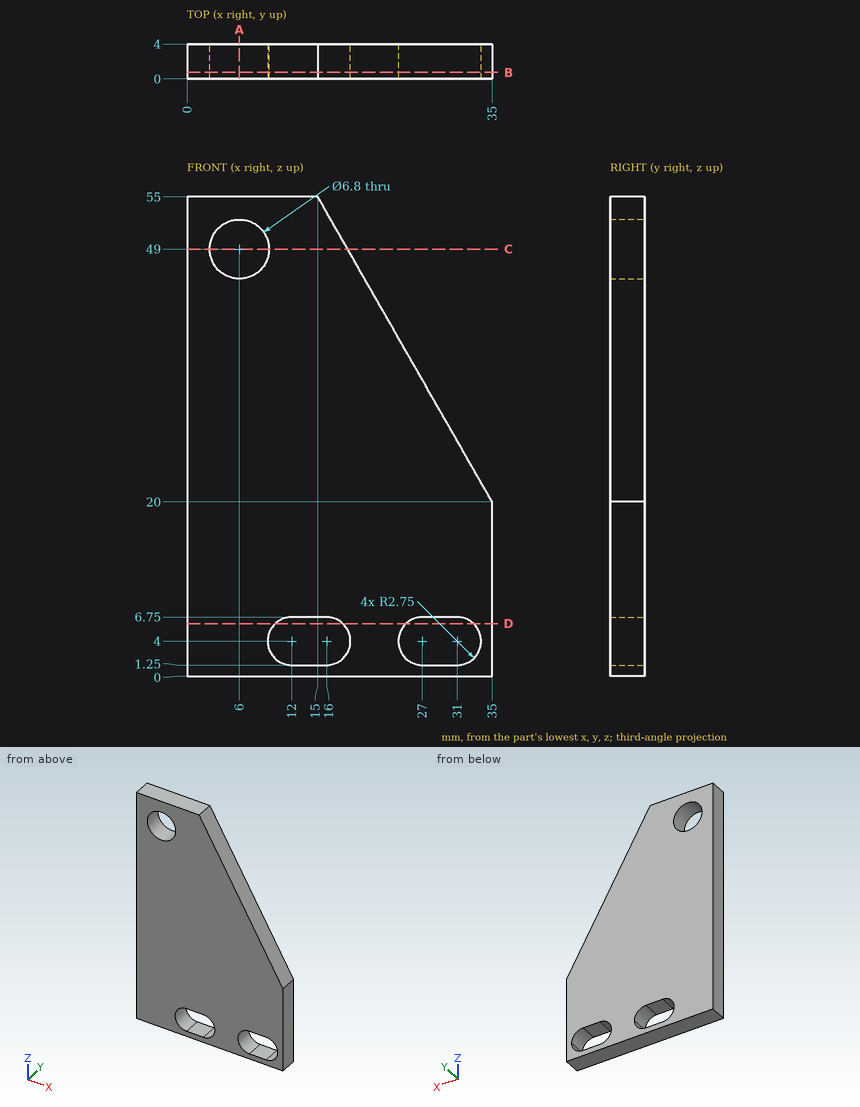
Here's the drawing with two shaded views (mm, measured from the low corner). I have some questions. Coordinates: 2 decimals unless noted, no trailing zeros. Order: outer loops, then holes, each group sorted by start corner. A loop starts at its lowest first (then second) coordinate and runs counter-clockwise, first axis right, second up. Notation, with made-up numbers: M 0.25,23.25 L 35.25,23.25 A22 ccw 35.25,46.25 Z; hole C 21.5,5 d8. An arc over 180 degrees is marked long. Answer as CSV lines item,"result".
Item 1: Imagine slicing it at A-A on x = 6. Write out the boundary of the cut face in (y, z), plus the area to 3 significant figures.
Results found:
outline,"M 0,0 L 4,0 L 4,45.6 L 0,45.6 Z; M 0,52.4 L 4,52.4 L 4,55 L 0,55 Z"
area,"193 mm2"
Item 2: Imagine slicing it at C-C on z = 49. Write out the boundary of the cut face in (x, y).
Results found:
outline,"M 0,0 L 2.6,0 L 2.6,4 L 0,4 Z; M 9.4,0 L 18.43,0 L 18.43,4 L 9.4,4 Z"
Item 3: Imagine slicing it at D-D on z = 6. Write out the boundary of the cut face in (x, y).
Results found:
outline,"M 0,0 L 10.11,0 L 10.11,4 L 0,4 Z; M 17.89,0 L 25.11,0 L 25.11,4 L 17.89,4 Z; M 32.89,0 L 35,0 L 35,4 L 32.89,4 Z"
Item 4: For pin 1 (1 mm diameter, centred on x = 20.5, y = 1.5, fed in from +Z); pin 2 (4 mm diameter, centred on x = 6, z = 49, fed in from +Y), each with a flat end and sliding along its axis, tell me the tip position at first contact or that it passes through.
Results found:
pin 1,"z = 46.25"
pin 2,"through"
Item 5: Imagine slicing it at B-B on y = 0.75. Write out the boundary of the cut face in (x, z).
Results found:
outline,"M 0,0 L 35,0 L 35,20 L 15,55 L 0,55 Z; hole C 6,49 d6.8; hole M 12,1.25 L 16,1.25 A2.75 ccw 16,6.75 L 12,6.75 A2.75 ccw Z; hole M 27,1.25 L 31,1.25 A2.75 ccw 31,6.75 L 27,6.75 A2.75 ccw Z"
Item 6: If I drill on line 1 (Z direction, x = 6, y = 1.5); line 2 (X direction, y = 1.45, z = 2); line 3 (Z direction, x = 33, y = 2.6), over which ranges is the centre line in solid material (lowest first)?
Results found:
line 1,"0 to 45.6, 52.4 to 55"
line 2,"0 to 10.11, 17.89 to 25.11, 32.89 to 35"
line 3,"0 to 2.11, 5.89 to 23.5"
